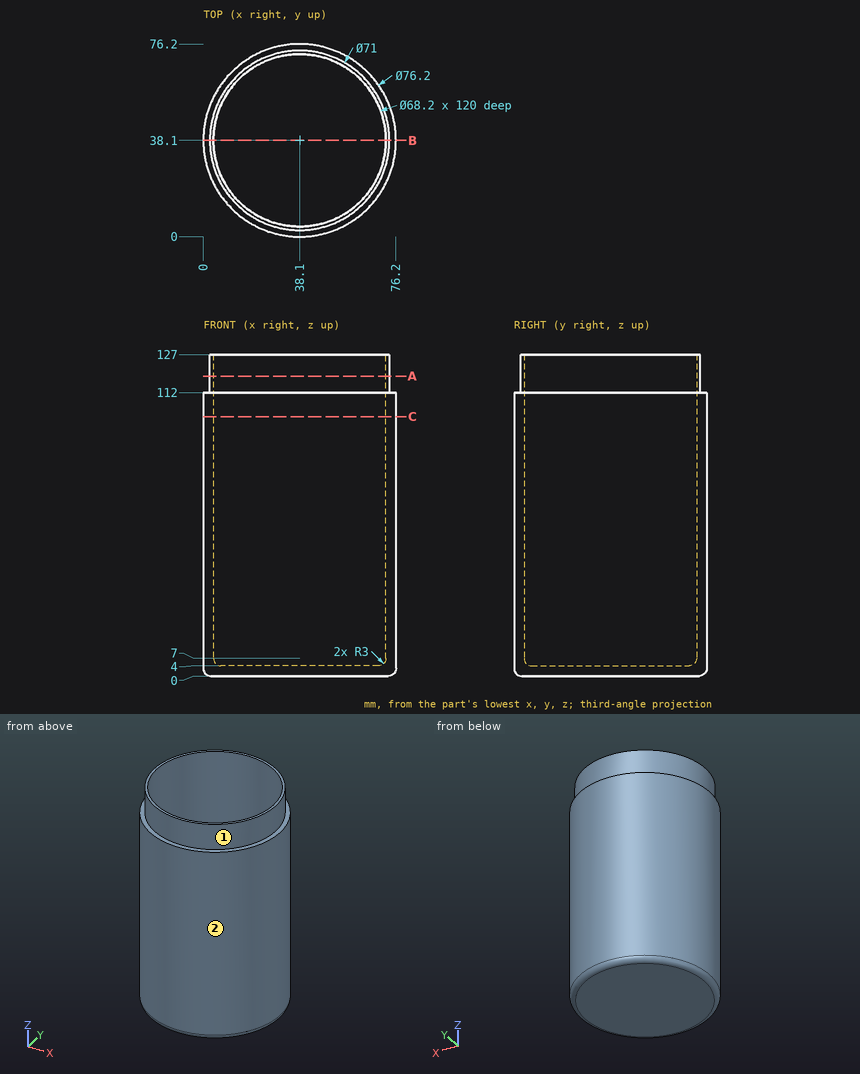
Check sheet for the drawn part. Datum: minimum x, y, z corner. Units: mm. A direction names the side the tool comes from. Give positions to 0.01 mm unless a question says otherwise; leave off trailing zeros. Loops run counter-clockwise (first coordinate to the right, second up) from the corner with the lowest first, then second, coordinate; pieces in that order, holes last.
1) Thickness scan on line 1 along Y through (x, z) = (38.1, 55.5); line 2 along Y through (x, z) = (14, 90). Record the ranges inside material, lowest first.
2) Set-up check for the marked faces 1 and 2: record each of +Z, -Z, +X, -X, +Y, -Y from which the full face is reachable in a straight line by a thin tool's end or side.
3) Depth check by flat-ended pin: pin 1 Ø2 at (x, y) = (21.5, 24.5) entering from +Z; pin 2 Ø2 at (y, z) = (26, 109) entering from -X; pin 3 Ø2 at (x, y) = (57.5, 50.5) entering from -Z; pin 4 Ø5 at (x, z) = (15, 62) entering from -Y. Enter the tip coordinate at first touch or a pass-through.
4) Sectioned sample at C-C, the plane z = 102.5. Enter the section's corners in (x, y).
5) Sectioned sample at A-A, the plane z = 118.5. Enter the section's corners in (x, y).
6) Sectioned sample at B-B, the plane y = 38.1. Enter the section's corners in (x, z).
Answers:
1. line 1: y = 0 to 4, 72.2 to 76.2
1. line 2: y = 8.59 to 13.98, 62.22 to 67.61
2. face 1: +Z
2. face 2: +Z, -Z
3. pin 1: stops at z = 4
3. pin 2: stops at x = 1.65
3. pin 3: stops at z = 0
3. pin 4: stops at y = 6.05
4. outline: circle Ø76.2 at (38.1, 38.1); hole circle Ø68.2 at (38.1, 38.1)
5. outline: circle Ø71 at (38.1, 38.1); hole circle Ø68.2 at (38.1, 38.1)
6. outline: (0, 3) arc R3 ccw to (3, 0) - (73.2, 0) arc R3 ccw to (76.2, 3) - (76.2, 112) - (73.6, 112) - (73.6, 127) - (72.2, 127) - (72.2, 7) arc R3 cw to (69.2, 4) - (7, 4) arc R3 cw to (4, 7) - (4, 127) - (2.6, 127) - (2.6, 112) - (0, 112) - close
